The model under review builds one solid part; all positions refer to its coordinate system, in mm. Face numbers are marked on the shaded views. A direction names the side the tool comes from. Round coordinates to 2 decimals unless told otherwise and drop trailing zeros. Order: outer loops, then holes, each group sorted by start corner. A loop starts at its lowest first (then second) coordinate and runs counter-clockwise, first axis right, second up. Notation, with made-up numbers: M -28,-6.5 L -18,-6.5 A8 cw -18,-0.5 Z; hole C 48.5,-20 d5. An arc over 180 degrees is marked long. Answer as a JSON object with one key per item and string values. Group by question number.
1) Consider section C-C, the plane x = -31. Write out the cut boundary in (y, z), then the cut area to 3 significant figures.
2) Consider section B-B, the plane y = 47.5. Write out the cut boundary in (x, z).
3) Insertion check: pin 1 Ø5 at (y, z) = (24.5, -5) entering from -X; pin 2 Ø5 at (x, z) = (-13.5, -1) entering from +Y; pin 3 Ø12 at (x, y) = (-31.5, 56) entering from -Z. Each pin has a flat end and moves straight along its axis. Give the tip position at first contact, or say it passes through.
4) The part is to be moulded in two halves that separate along Y. For the marked faces 1, 2 and 3, say which applies: +Y half, -Y half, draft (parallel to the pull), parting line (faces both ways), or undercut.
5) For the marked faces 4, 5 and 6, list the 3-axis set-ups (+Z, -Z, +X, -X, +Y, -Y) from which the entire face can be reached by the end or side of a thin tool; tool diameter is ignored.
6) Consider section A-A, the plane z = 1.75. Write out the cut boundary in (x, y), then the cut area to 3 significant figures.
7) Consider section D-D, the plane x = -24. Write out the cut boundary in (y, z).
8) To check wall thickness, follow line 1 (Z direction, x = -23.5, y = 55.5); line 2 (Y direction, x = -36.5, z = 0.75); line 3 (X direction, y = 48, z = 1.75). State the ranges of each line that lie inside material, in increasing order.
```python
from build123d import *

# Parameters (mm, degrees)
CROQUIS1_R                 = 8
SALIENTE_EXTRUIR1_DEPTH    = 8
SALIENTE_EXTRUIR2_DEPTH    = 3
CORTAR_EXTRUIR1_DEPTH      = 10
CORTAR_EXTRUIR1_DEPTH_BACK = 10


with BuildPart() as part:
    # Croquis1 → Saliente-Extruir1 (new body)
    with BuildSketch(Plane.XY):
        with Locations((-35.87588422, 30.387347076)):
            Circle(CROQUIS1_R)
    extrude(amount=-SALIENTE_EXTRUIR1_DEPTH)

    # Croquis2 → Saliente-Extruir2 (add)
    with BuildSketch(Plane.XY):
        with BuildLine():
            Line((-33.848986828, 60.448524076), (-45.879424714, 41.56451924))
            Line((-45.879424714, 41.56451924), (-50.233521284, 34.729956653))
            ThreePointArc((-50.233521284, 34.729956653), (-50.520324327, 27.140752867), (-47.053056384, 20.383806582))
            Line((-47.053056384, 20.383806582), (-40.218493797, 16.029710012))
            ThreePointArc((-40.218493797, 16.029710012), (-32.629290011, 15.74290697), (-25.872343726, 19.210174912))
            Line((-25.872343726, 19.210174912), (-21.518247156, 26.044737499))
            Line((-21.518247156, 26.044737499), (-9.48780927, 44.928742335))
            ThreePointArc((-9.48780927, 44.928742335), (-8.42457278, 50.958656113), (-11.93654397, 55.974270768))
            Line((-11.93654397, 55.974270768), (-13.952719889, 57.258716487))
            Line((-13.952719889, 57.258716487), (-20.787282476, 61.612813057))
            Line((-20.787282476, 61.612813057), (-22.803458395, 62.897258775))
            ThreePointArc((-22.803458395, 62.897258775), (-28.833372173, 63.960495266), (-33.848986828, 60.448524076))
        make_face()
    extrude(amount=SALIENTE_EXTRUIR2_DEPTH)

    # Croquis5 → Cortar-Extruir1 (cut, two sides)
    with BuildSketch(Plane.XY) as cortar_extruir1_sk:
        Polygon((-19.390525704, 46.02780209), (-21.002424529, 43.497627753), (-30.279730433, 49.407923445), (-28.667831608, 51.938097782), align=None)
        Polygon((-30.431281855, 28.697286399), (-32.04318068, 26.167112062), (-41.320486584, 32.077407754), (-39.708587759, 34.607582091), align=None)
    extrude(amount=CORTAR_EXTRUIR1_DEPTH, mode=Mode.SUBTRACT)
    extrude(cortar_extruir1_sk.sketch, amount=-CORTAR_EXTRUIR1_DEPTH_BACK, mode=Mode.SUBTRACT)


solid = part.part
```
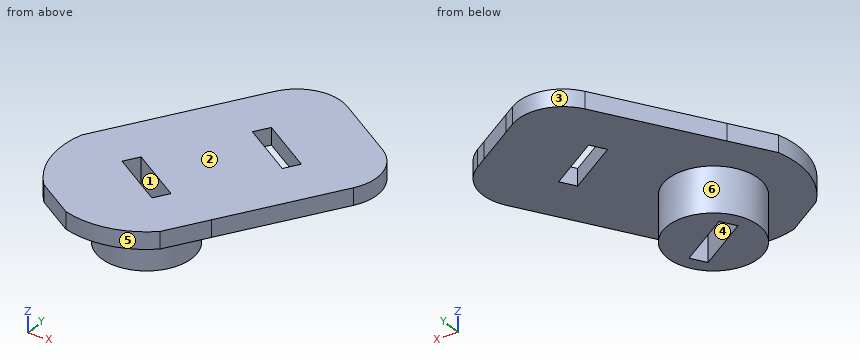
Results list:
{
 "1": {"outline": "M 16.2,0 L 24.04,0 L 24.04,-8 L 27.8,-8 L 27.8,3 L 16.2,3 Z; M 29.06,-8 L 36.73,-8 L 36.73,0 L 63.14,0 L 63.14,3 L 29.06,3 Z", "area": "228 mm^2"},
 "2": {"outline": "M -42.1,0 L -27.28,0 L -27.28,3 L -42.1,3 Z; M -21.7,0 L -8.42,0 L -8.42,3 L -21.7,3 Z"},
 "3": {"pin 1": "x = -43.12", "pin 2": "y = 58.43", "pin 3": "z = 0"},
 "4": {"face 1": "undercut", "face 2": "draft", "face 3": "+Y half"},
 "5": {"face 4": "+Z, -Z", "face 5": "+Z, -Z, -Y", "face 6": "-Z"},
 "6": {"outline": "M -50.23,34.73 A15 ccw -47.05,20.38 L -40.22,16.03 A15 ccw -25.87,19.21 L -9.49,44.93 A8 ccw -11.94,55.97 L -22.8,62.9 A8 ccw -33.85,60.45 Z; hole M -41.32,32.08 L -32.04,26.17 L -30.43,28.7 L -39.71,34.61 Z; hole M -30.28,49.41 L -21,43.5 L -19.39,46.03 L -28.67,51.94 Z", "area": "1,250 mm^2"},
 "7": {"outline": "M 22.15,0 L 45.41,0 L 45.41,3 L 22.15,3 Z; M 48.96,0 L 63.52,0 L 63.52,3 L 48.96,3 Z"},
 "8": {"line 1": "0 to 3", "line 2": "15.4 to 29.01, 32.56 to 56.29", "line 3": "-41.78 to -28.07, -22.49 to -8.33"}
}
